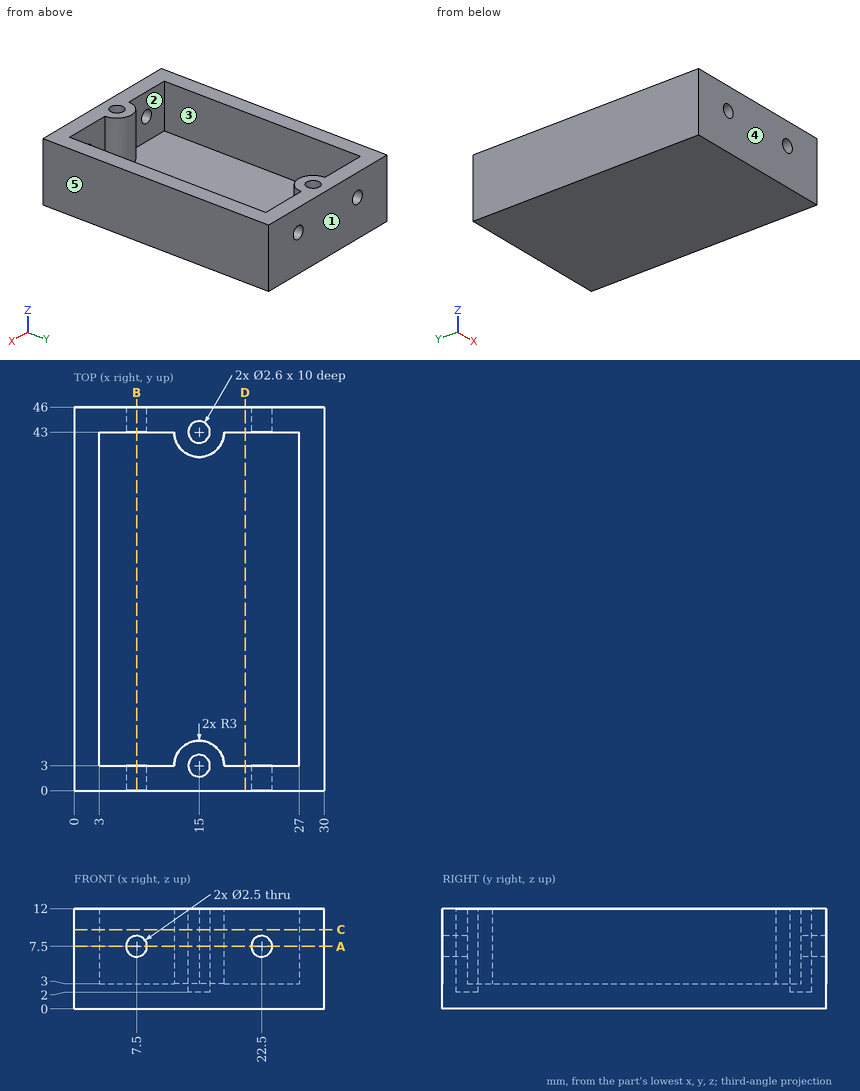
Check sheet for the drawn part. Datum: minimum x, y, z corner. Units: mm. A direction names the side the tool comes from. Round coordinates to 2 decimals unless told otherwise and drop trailing zeros. Loops run counter-clockwise (first coordinate to the right, second up) from the corner with the lowest first, then second, coordinate; pieces in that order, holes last. Notation, with made-up numbers: M 66.5,40.25 L 115.5,40.25 A12 cw 115.5,62.25 Z; hole C -15,46 d10. An arc over 180 degrees is marked long. One line per question, with ' | ' between items. Start each with the question number.
Item 1: Release check for a two-part mould opening along Y. For the marked faces 3, 4 and 5 record: released by +Y, released by -Y, zero draft, split by the parting line, or undercut.
Item 2: Gauge pin test, flat ends, axial feed: pin 1 Ø2.5 at (x, y) = (15, 43) entering from +Z; pin 2 Ø2 at (x, z) = (7.5, 7.5) entering from +Y. Record the tip position at first contact, or that the pin passes through.
Item 3: Section check B-B (x = 7.5). Record the boundary of the cut face in (y, z), and give its area (3 significant figures).
Item 4: Section check D-D (x = 20.5). Record the boundary of the cut face in (y, z), and give its area (3 significant figures).
Item 5: Set-up check for the marked faces 1 and 2: record each of +Z, -Z, +X, -X, +Y, -Y from which the full face is reachable in a straight line by a thin tool's end or side.
Item 6: Scan lines: probe 1 along Y at (x, z) = (15, 5); probe 2 along X at (y, z) = (23, 8); probe 3 along Y at (x, z) = (23.5, 10.5). Record each from-to range of solid material in increasing order.
Item 7: Section check C-C (z = 9.5). Record the boundary of the cut face in (x, y), and give its area (3 significant figures).
Item 8: Section check A-A (z = 7.5). State how many separate pieces and enclosed holes the cut face has, and give its area (3 significant figures).
Worked out:
1) face 3: undercut | face 4: released by -Y | face 5: zero draft
2) pin 1: z = 2 | pin 2: through
3) outline: M 0,0 L 46,0 L 46,6.25 L 43,6.25 L 43,3 L 3,3 L 3,6.25 L 0,6.25 Z; M 0,8.75 L 3,8.75 L 3,12 L 0,12 Z; M 43,8.75 L 46,8.75 L 46,12 L 43,12 Z | area: 177 mm^2
4) outline: M 0,0 L 46,0 L 46,12 L 43,12 L 43,3 L 3,3 L 3,12 L 0,12 Z | area: 192 mm^2
5) face 1: +Z, -Z, +X, -X, +Y | face 2: +Z
6) probe 1: 0 to 1.7, 4.3 to 6, 40 to 41.7, 44.3 to 46 | probe 2: 0 to 3, 27 to 30 | probe 3: 0 to 3, 43 to 46
7) outline: M 0,0 L 30,0 L 30,46 L 0,46 Z; hole M 3,3 L 12,3 A3 cw 18,3 L 27,3 L 27,43 L 18,43 A3 cw 12,43 L 3,43 Z; hole C 15,3 d2.6; hole C 15,43 d2.6 | area: 438 mm^2
8) separate pieces: 4 | enclosed holes: 2 | area: 408 mm^2
